CAD build for the part. Positions are in the model's coordinates, mm. A direction names the side the tool comes from. Coordinates: 2 decimals unless noted, no trailing zeros. Loops run counter-clockwise (first coordinate to the right, second up) from the corner with the lowest first, then second, coordinate; pieces in that order, holes last. Notation, with made-up numbers: (78, -0.5) -> (130, -0.5) arc R22 cw to (130, 29.5) -> close; hole circle Ø7 at (78, 50.5). An arc over 180 degrees is marked (long way). Write each question's results on one line, items separated by ' | '.
```python
from build123d import *

# Parameters (mm, degrees)
SKETCH_R    = 1
PAD_DEPTH   = 12.5
BOX_W       = 19
BOX_H       = 19
BOX_DEPTH   = 19
SKETCH001_R = 1.5
HOLE_DEPTH  = 2.001
FILLET_R    = 3


with BuildPart() as part:
    # Sketch → Pad (new body, symmetric)
    with BuildSketch(Plane.XZ):
        with BuildLine():
            Line((0, 0), (-16, 0))
            Line((-16, 0), (-16, 12))
            ThreePointArc((-13.588072, 15.157725), (-17.986745, 16.017512), (-16, 12))
            Line((-13.588072, 15.157725), (-10, 2))
            Line((-10, 2), (0, 2))
            Line((0, 2), (0, 0))
        make_face()
        with Locations((-16, 14.5)):
            Circle(SKETCH_R, mode=Mode.SUBTRACT)
    extrude(amount=PAD_DEPTH, both=True)

    # Box → Box (cut)
    with BuildSketch(Plane(origin=(-7, 9.5, 2), x_dir=(-1, 0, 0), z_dir=(0, 0, 1))):
        with Locations((9.5, 9.5)):
            Rectangle(BOX_W, BOX_H)
    extrude(amount=BOX_DEPTH, mode=Mode.SUBTRACT)

    # Sketch001 (on Face14 of Box) → Hole (cut, through all)
    with BuildSketch(Plane(origin=(-7, 9.5, 2), x_dir=(-1, 0, 0), z_dir=(0, 0, 1))):
        with Locations((5, 9.5)):
            Circle(SKETCH001_R)
        with Locations((-2, 16.5)):
            Circle(SKETCH001_R)
        with Locations((-2, 2.5)):
            Circle(SKETCH001_R)
    extrude(amount=-HOLE_DEPTH, mode=Mode.SUBTRACT)

    # Fillet
    fillet_edges = [part.edges().sort_by_distance(p)[0] for p in [
        (0, 12.5, 1),
        (0, -12.5, 1),
    ]]
    fillet(fillet_edges, radius=FILLET_R)


solid = part.part
```
Q1. Cut at A-A on y = 7. Write the cut outline in (x, z).
Results are:
outline: (-16, 0) -> (-6.5, 0) -> (-6.5, 2) -> (-16, 2) -> close; (-3.5, 0) -> (0, 0) -> (0, 2) -> (-3.5, 2) -> close
Q2. Drop flat-ended pins along their axis: pin 1 (1 mm diameter, centred on y = 8.5, z = 9.5, fed in from +X); pin 2 (9.5 mm diameter, centred on y = 4, z = 3.5, fed in from -X); pin 3 (1 mm diameter, centred on x = -7.5, y = -7, fed in from +Z); pin 4 (2.5 mm diameter, centred on x = -16, z = 14.5, fed in from -Y). Give the stop position or say it passes through.
Results are:
pin 1: through | pin 2: x = -16 | pin 3: z = 2 | pin 4: y = -12.5
Q3. Cut at D-D on y = 10.5. Write the cut outline in (x, z), and give its area (3 significant figures).
Results are:
outline: (-16, 0) -> (-0.17, 0) -> (-0.17, 2) -> (-10, 2) -> (-13.59, 15.16) arc R2.5 ccw (long way) to (-16, 12) -> close; hole circle Ø2 at (-16, 14.5) | area: 97.0 mm^2
Q4. Which spindle directions (+Z, -Z, +X, -X, +Y, -Y) get a long thin tool onto all of the face, cutting with end or side? Do faces 5 (the flat face through (-11.82, -11.02, 8.67)), 6 (the flat face through (-14, 9.5, 9)), 7 (the flat face through (-16, 0, 1)), 8 (the flat face through (-8, 0, 2)). Say none if no direction does.
Results are:
face 5: +Z, +X, +Y, -Y | face 6: +Z, +X, -X | face 7: -Z, -X, +Y, -Y | face 8: +Z, +X
Q5. Pull direction X, two halves, no side cores. Call faces 1 (the cylindrical face through (-5.69, 8.33, 1.01)), 2 (the cylindrical face through (-0.86, -11.6, 0.99)), 3 (the cylindrical face through (-18, -11, 16)), 4 (the cylindrical face through (-15.54, -10.98, 13.61)): +X half, -X half, draft (parallel to the pull), parting line (faces both ways), or undercut.
Results are:
face 1: undercut | face 2: +X half | face 3: parting line | face 4: undercut
Q6. Wall check: L1, parallel to Y at x = -5, z = 0.9; L2, parallel to X at y = -7, z = 0.45; L3, parallel to X at y = 0, z = 0.9. Give the ranges that are in metal, low to high. Write a range as from..to.
Results are:
L1: -12.5..-8.5, -5.5..5.5, 8.5..12.5 | L2: -16..-6.5, -3.5..0 | L3: -16..-13.5, -10.5..0
Q7. Cut at B-B on z = 9.5. Write the cut outline in (x, y).
Results are:
outline: (-16, -12.5) -> (-12.05, -12.5) -> (-12.05, -9.5) -> (-16, -9.5) -> close; (-16, 9.5) -> (-12.05, 9.5) -> (-12.05, 12.5) -> (-16, 12.5) -> close
Q8. Cut at C-C on z = 14.5. Write the cut outline in (x, y).
Results are:
outline: (-18.5, -12.5) -> (-17, -12.5) -> (-17, -9.5) -> (-18.5, -9.5) -> close; (-18.5, 9.5) -> (-17, 9.5) -> (-17, 12.5) -> (-18.5, 12.5) -> close; (-15, -12.5) -> (-13.41, -12.5) -> (-13.41, -9.5) -> (-15, -9.5) -> close; (-15, 9.5) -> (-13.41, 9.5) -> (-13.41, 12.5) -> (-15, 12.5) -> close
